The figure shows three views and two pictorial views of one solid part (mm, origin at its lowest corner). Answer the questions. A direction names the side the tool comes from. Coordinates: 2 decimals unless noted, no trailing zeros. Loops run counter-clockwise (first coordinate to the right, second up) from the corner with the lowest first, then second, coordinate; pieces in that order, holes last. Notation, with made-up numbers: (-28, 13.25) -> (-1, 13.25) arc R6 cw to (-1, 17.25) -> close; hole circle Ø4 at (22, -14.75). An arc over 180 degrees is marked (long way). Use a Markdown table: item, result. Add a question column.
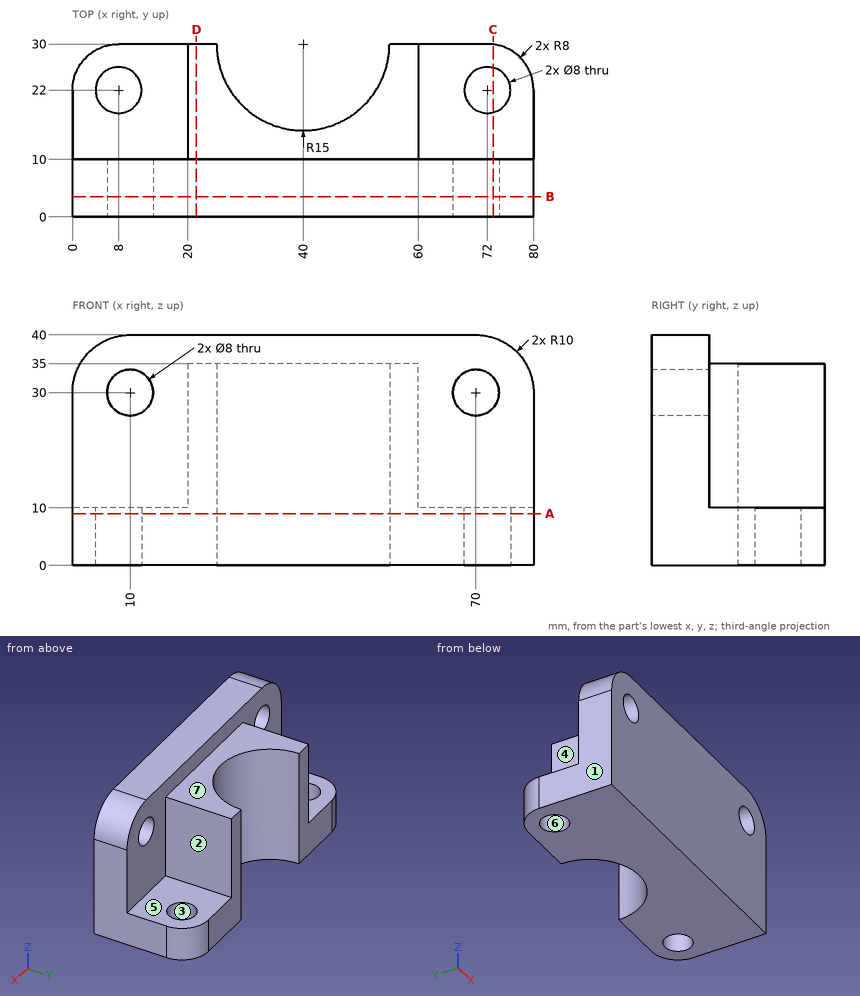
Item 1: Section C-C (x = 73) is taken. Determine the outline of the cut face in (y, z), then the cut area to 3 significant figures.
Item 2: For a pull along X with two mould halves and no side action, classify the marked faces 1, 2 and 3 as +X half, -X half, draft (parallel to the pull), parting line (faces both ways), or undercut.
Item 3: For the marked faces 4, 5, 6 and 7, determine the directions among +Z, -Z, +X, -X, +Y, -Y from which every point of the face is accessible in a straight line to the end or side of a thin tool.
Item 4: Given pin 1 (7 mm diameter, centred on x = 70, z = 30, fed in from +Y); pin 2 (1.5 mm diameter, centred on y = 16, z = 14.5, fed in from +X); pin 3 (10 mm diameter, centred on x = 29, y = 26, fed in from +Z); pin 4 (9 mm diameter, centred on x = 8, y = 22, fed in from +Z), each flat-ended and moving along its own axis, determine where each tip first touches the part or whether it passes through.
Item 5: Section A-A (z = 9) is taken. Determine the outline of the cut face in (x, y), then the cut area to 3 significant figures.
Item 6: Section D-D (x = 21.5) is taken. Determine the outline of the cut face in (y, z).
Item 7: Find the intervals of material crossed by probe 1 along Y at (x, z) = (8, 3); probe 2 along Y at (x, z) = (61, 21), in increasing order.
Item 8: Section B-B (y = 3.5) is taken. Determine the outline of the cut face in (x, z).
Output:
| question | item | result |
|---|---|---|
| 1 | outline | (0, 0) -> (18.13, 0) -> (18.13, 10) -> (10, 10) -> (10, 27.35) -> (0, 27.35) -> close; (0, 32.65) -> (10, 32.65) -> (10, 39.54) -> (0, 39.54) -> close; (25.87, 0) -> (29.94, 0) -> (29.94, 10) -> (25.87, 10) -> close |
| 1 | area | 464 mm2 |
| 2 | face 1 | -X half |
| 2 | face 2 | +X half |
| 2 | face 3 | undercut |
| 3 | face 4 | +Z, -X, +Y |
| 3 | face 5 | +Z, +X, +Y |
| 3 | face 6 | +Z, -Z |
| 3 | face 7 | +Z, +X, -X, +Y |
| 4 | pin 1 | passes through |
| 4 | pin 2 | stops at x = 60 |
| 4 | pin 3 | stops at z = 35 |
| 4 | pin 4 | stops at z = 10 |
| 5 | outline | (0, 0) -> (80, 0) -> (80, 22) arc R8 ccw to (72, 30) -> (55, 30) arc R15 cw to (25, 30) -> (8, 30) arc R8 ccw to (0, 22) -> close; hole circle Ø8 at (8, 22); hole circle Ø8 at (72, 22) |
| 5 | area | 1,920 mm2 |
| 6 | outline | (0, 0) -> (30, 0) -> (30, 35) -> (10, 35) -> (10, 40) -> (0, 40) -> close |
| 7 | probe 1 | y = 0 to 18, 26 to 30 |
| 7 | probe 2 | y = 0 to 10 |
| 8 | outline | (0, 0) -> (80, 0) -> (80, 30) arc R10 ccw to (70, 40) -> (10, 40) arc R10 ccw to (0, 30) -> close; hole circle Ø8 at (10, 30); hole circle Ø8 at (70, 30) |
